Design review of the part built by this model. Coordinates are the model's own, in mm. A direction names the side the tool comes from. Give positions to 0.01 mm unless a question says otherwise; leave off trailing zeros. Loops run counter-clockwise (first coordinate to the right, second up) from the corner with the lowest first, then second, coordinate; pieces in that order, holes last. Notation, with made-up numbers: M 83.5,47 L 141.5,47 A12 ccw 141.5,52 Z; hole C 33,18 d3. An arc over 180 degrees is marked long. Answer as CSV lines item,"result".
```python
from build123d import *


with BuildPart() as f2:
    # F2: sweep along a path in F0
    with BuildLine(Plane.XY) as f2_path:
        Line((0, 399.9603311834), (0, -399.9603311834))
    # F1 (on Front) → F2 (sweep)
    with BuildSketch(Plane.XZ):
        Polygon((20, -40), (20, 0), (-20, 0), (-20, -3.175), (16.825, -3.175), (16.825, -40), align=None)
    sweep(path=f2_path.line)


solid = f2.part
```
1. We need section A-A, the plane y = 271. Write out the cut boundary in (x, z) (3 decimals), plus the area to 3 significant figures.
Answer block:
outline,"M -20,-3.175 L 16.825,-3.175 L 16.825,-40 L 20,-40 L 20,0 L -20,0 Z"
area,"244 mm²"
2. We need section C-C, the plane x = 0.5. Write out the cut boundary in (y, z) (3 decimals), plus the area to 3 significant figures.
Answer block:
outline,"M -399.96,-3.175 L 399.96,-3.175 L 399.96,0 L -399.96,0 Z"
area,"2,540 mm²"
3. We need section B-B, the plane z = -28.5. Write out the cut boundary in (x, y) (3 decimals), plus the area to 3 significant figures.
Answer block:
outline,"M 16.825,-399.96 L 20,-399.96 L 20,399.96 L 16.825,399.96 Z"
area,"2,540 mm²"
4. For faces 1 (the flat face through (20, -6, -20)), 2 (the flat face through (16.825, -6, -21)), list the 3-axis set-ups (+Z, -Z, +X, -X, +Y, -Y) from which the entire face can be reached by the end or side of a thin tool; tool diameter is ignored.
Answer block:
face 1,"+Z, -Z, +X, +Y, -Y"
face 2,"-Z, -X, +Y, -Y"
5. To check wall thickness, follow L1, parallel to X at y = -152.5, z = -22.5 (3 decimals); L2, parallel to Z at x = -7, y = -49.5 (3 decimals). State the ranges of each line that lie inside material, in increasing order. Write a range as [from, to].
Answer block:
L1,"[16.825, 20]"
L2,"[-3.175, 0]"
6. For P1, Ø1, axis at x = 4, y = -7.5, coming from the -Z side (3 decimals); P2, Ø5, axis at y = 75, z = -25.5, coming from the -X side (3 decimals); P3, Ø6, axis at x = 12.5, z = -28, coming from the -Y side, all flat-tipped, find the tip position at first contact; note any pin that passes through.
Answer block:
P1,"z = -3.175"
P2,"x = 16.825"
P3,"through"
